Geometry check sheet. Reference: drawing and pictorial views, mm from the part's lowest x, y, z. A direction names the side the tool comes from. Round coordinates to 2 decimals unless told otherwise and drop trailing zeros. Write each loop counter-clockwise with the first axis right and the second up, starting at its lowest first coordinate (ties: lowest second). Pieces come first, ordered by that corner, then holes.
Item 1: Section check C-C, the plane y = 3.75. Record the cut outline in (x, z).
Item 2: Section check B-B, the plane x = 65. Record the cut outline in (y, z), plus the area to 3 significant figures.
Item 3: Section check D-D, the plane y = 7.5. Record the cut outline in (x, z).
Item 4: Material ranges on line 1 along Y through (x, z) = (85, 0.5); line 2 along Y through (x, z) = (79, 2.5); line 3 along Z through (x, y) = (9.5, 7.25), recorded low to high.
Item 5: Section check A-A, the plane z = 10.75. Record the cut outline in (x, y), plus the area to 3 significant figures.
Item 6: Release check for a two-part mould opening along Y. For the marked faces 3, 4 and 5 record: pulls with the +Y half, pulls with the -Y half, needs draft (parallel to the pull), parting line crosses it, or undercut.
Item 7: Depth check by flat-ended pin: pin 1 (8 mm diameter, centred on y = 6.5, z = 8, fed in from -X). Enter the tip coordinate at first touch or a pass-through.
Item 8: Set-up check for the marked faces 1 and 2: record each of +Z, -Z, +X, -X, +Y, -Y from which the full face is reachable in a straight line by a thin tool's end or side.
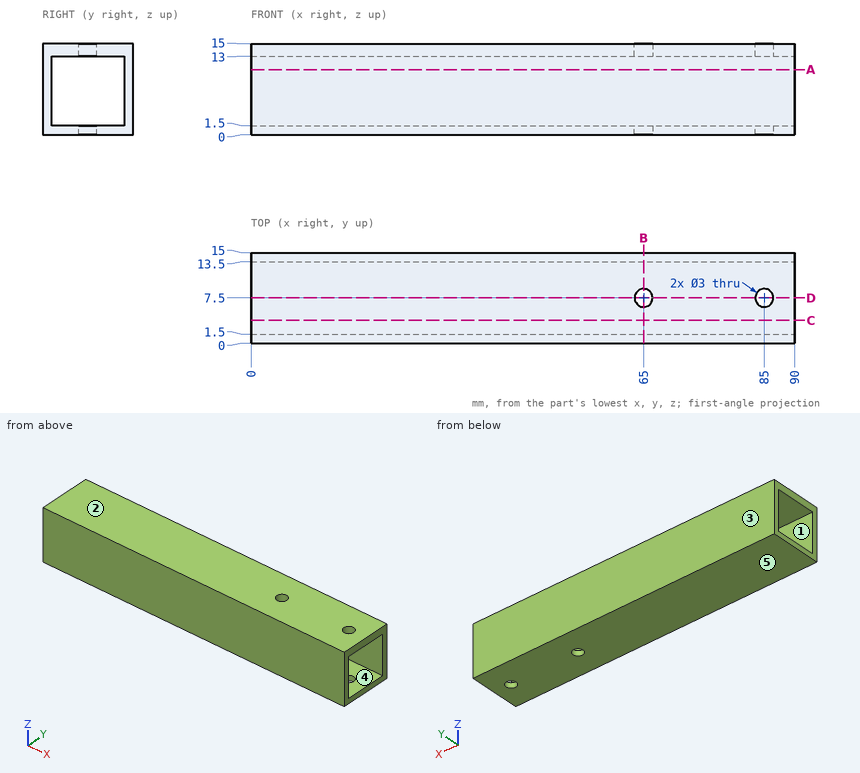
Values found:
1. outline: (0, 0) - (90, 0) - (90, 1.5) - (0, 1.5) - close; (0, 13) - (90, 13) - (90, 15) - (0, 15) - close
2. outline: (0, 0) - (6, 0) - (6, 1.5) - (1.5, 1.5) - (1.5, 13) - (6, 13) - (6, 15) - (0, 15) - close; (9, 0) - (15, 0) - (15, 15) - (9, 15) - (9, 13) - (13.5, 13) - (13.5, 1.5) - (9, 1.5) - close
2. area: 76.5 mm2
3. outline: (0, 0) - (63.5, 0) - (63.5, 1.5) - (0, 1.5) - close; (0, 13) - (63.5, 13) - (63.5, 15) - (0, 15) - close; (66.5, 0) - (83.5, 0) - (83.5, 1.5) - (66.5, 1.5) - close; (66.5, 13) - (83.5, 13) - (83.5, 15) - (66.5, 15) - close; (86.5, 0) - (90, 0) - (90, 1.5) - (86.5, 1.5) - close; (86.5, 13) - (90, 13) - (90, 15) - (86.5, 15) - close
4. line 1: y = 0 to 6, 9 to 15
4. line 2: y = 0 to 1.5, 13.5 to 15
4. line 3: z = 0 to 1.5, 13 to 15
5. outline: (0, 0) - (90, 0) - (90, 1.5) - (0, 1.5) - close; (0, 13.5) - (90, 13.5) - (90, 15) - (0, 15) - close
5. area: 270 mm2
6. face 3: pulls with the +Y half
6. face 4: undercut
6. face 5: needs draft
7. pin 1: passes through
8. face 1: +X, -X
8. face 2: +Z, +X, -X, +Y, -Y
